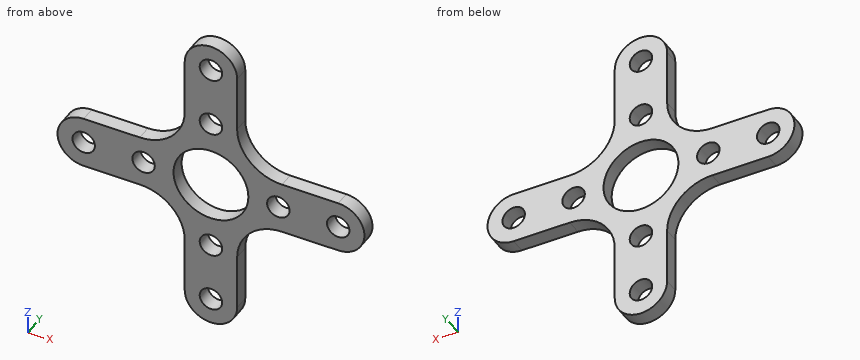
```python
from build123d import *

# Parameters (mm, degrees)
BOSS_EXTRUDE1_DEPTH = 2
SKETCH2_R           = 1.5
SKETCH2_R_2         = 5
CUT_EXTRUDE1_DEPTH  = 2


with BuildPart() as part:
    # Sketch1 → Boss-Extrude1 (new body)
    with BuildSketch(Plane(origin=(0, 0, 0), x_dir=(1, 0, 0), z_dir=(0, 1, 0))):
        with BuildLine():
            Line((-3.5, 17), (-3.5, 9.5))
            ThreePointArc((-3.5, 9.5), (-5.257359313, 5.257359313), (-9.5, 3.5))
            Line((-9.5, 3.5), (-17, 3.5))
            ThreePointArc((-17, 3.5), (-20.5, 0), (-17, -3.5))
            Line((-17, -3.5), (-9.5, -3.5))
            ThreePointArc((-9.5, -3.5), (-5.257359313, -5.257359313), (-3.5, -9.5))
            Line((-3.5, -9.5), (-3.5, -17))
            ThreePointArc((-3.5, -17), (0, -20.5), (3.5, -17))
            Line((3.5, -17), (3.5, -9.5))
            ThreePointArc((3.5, -9.5), (5.257359313, -5.257359313), (9.5, -3.5))
            Line((9.5, -3.5), (17, -3.5))
            ThreePointArc((17, -3.5), (20.5, 0), (17, 3.5))
            Line((17, 3.5), (9.5, 3.5))
            ThreePointArc((9.5, 3.5), (5.257359313, 5.257359313), (3.5, 9.5))
            Line((3.5, 9.5), (3.5, 17))
            ThreePointArc((3.5, 17), (0, 20.5), (-3.5, 17))
        make_face()
    extrude(amount=BOSS_EXTRUDE1_DEPTH)

    # Sketch2 → Cut-Extrude1 (cut)
    with BuildSketch(Plane(origin=(0, 2, 0), x_dir=(1, 0, 0), z_dir=(0, 1, 0))):
        with Locations((0, 17)):
            Circle(SKETCH2_R)
        with Locations((0, 9)):
            Circle(SKETCH2_R)
        Circle(SKETCH2_R_2)
        with Locations((17, 0)):
            Circle(SKETCH2_R)
        with Locations((9, 0)):
            Circle(SKETCH2_R)
        with Locations((0, -17)):
            Circle(SKETCH2_R)
        with Locations((0, -9)):
            Circle(SKETCH2_R)
        with Locations((-17, 0)):
            Circle(SKETCH2_R)
        with Locations((-9, 0)):
            Circle(SKETCH2_R)
    extrude(amount=-CUT_EXTRUDE1_DEPTH, mode=Mode.SUBTRACT)


solid = part.part
```
Build history of the part. All positions in model axes, mm. Coordinates: 2 decimals unless noted, no trailing zeros. Order: outer loops, then holes, each group sorted by start corner. A loop starts at its lowest first (then second) coordinate and runs counter-clockwise, first axis right, second up.
Item 1: Drill centre lines: L1, parallel to Z at x = 0, y = 1.2; L2, parallel to Z at x = 17, y = 1.6. Where is each one in solid material? Low to high.
Filled in:
L1: z = -20.5 to -18.5, -15.5 to -10.5, -7.5 to -5, 5 to 7.5, 10.5 to 15.5, 18.5 to 20.5
L2: z = -3.5 to -1.5, 1.5 to 3.5
Item 2: Saw through at A-A on z = 0. List the corners of the cut face in (x, y), then the cut area to 3 significant figures.
Filled in:
outline: (-20.5, 0) - (-18.5, 0) - (-18.5, 2) - (-20.5, 2) - close; (-15.5, 0) - (-10.5, 0) - (-10.5, 2) - (-15.5, 2) - close; (-7.5, 0) - (-5, 0) - (-5, 2) - (-7.5, 2) - close; (5, 0) - (7.5, 0) - (7.5, 2) - (5, 2) - close; (10.5, 0) - (15.5, 0) - (15.5, 2) - (10.5, 2) - close; (18.5, 0) - (20.5, 0) - (20.5, 2) - (18.5, 2) - close
area: 38.0 mm2
Item 3: Drop flat-ended pins along their axis: pin 1 Ø0.6 at (y, z) = (1, 14) entering from -X; pin 2 Ø0.6 at (x, y) = (-14, 0.5) entering from -Z; pin 3 Ø1 at (x, y) = (11.5, 1) entering from +Z. Give the stop position or say it passes through.
Filled in:
pin 1: stops at x = -3.5
pin 2: stops at z = -3.5
pin 3: stops at z = 3.5
Item 4: Saw through at D-D on z = 9. List the corners of the cut face in (x, y), then the cut area to 3 significant figures.
Filled in:
outline: (-3.52, 0) - (-1.5, 0) - (-1.5, 2) - (-3.52, 2) - close; (1.5, 0) - (3.52, 0) - (3.52, 2) - (1.5, 2) - close
area: 8.08 mm2
Item 5: Saw through at C-C on x = 0. List the corners of the cut face in (y, z).
Filled in:
outline: (0, -20.5) - (2, -20.5) - (2, -18.5) - (0, -18.5) - close; (0, -15.5) - (2, -15.5) - (2, -10.5) - (0, -10.5) - close; (0, -7.5) - (2, -7.5) - (2, -5) - (0, -5) - close; (0, 5) - (2, 5) - (2, 7.5) - (0, 7.5) - close; (0, 10.5) - (2, 10.5) - (2, 15.5) - (0, 15.5) - close; (0, 18.5) - (2, 18.5) - (2, 20.5) - (0, 20.5) - close
Item 6: Saw through at B-B on y = 0.6. State how many separate pieces and enclosed holes the cut face has, then the cut area to 3 significant figures.
Filled in:
separate pieces: 1
enclosed holes: 9
area: 400 mm2
